from build123d import *

# Parameters (mm, degrees)
F0_R     = 1.55
F1_DEPTH = 1.5
F2_W     = 5
F2_H     = 2
F3_DEPTH = 1.5
F4_R     = 0.5
F5_DEPTH = 25
F7_DEPTH = 1.5
F8_R     = 3


with BuildPart() as f1:
    # F0 (on Right) → F1 (new body)
    with BuildSketch(Plane.YZ):
        with BuildLine():
            Line((-10, 0), (0, 0))
            Line((0, 0), (0, 30))
            Line((0, 30), (-10, 30))
            ThreePointArc((-10, 30), (-13.7334119498, 15), (-10, 0))
        make_face()
        with Locations((-10, 9.5)):
            Circle(F0_R, mode=Mode.SUBTRACT)
        with Locations((-6.5, 12.25)):
            Circle(F0_R, mode=Mode.SUBTRACT)
        with Locations((-10, 15)):
            Circle(F0_R, mode=Mode.SUBTRACT)
        with Locations((-10, 20.5)):
            Circle(F0_R, mode=Mode.SUBTRACT)
        with Locations((-6.5, 17.75)):
            Circle(F0_R, mode=Mode.SUBTRACT)
        with Locations((-3, 15)):
            Circle(F0_R, mode=Mode.SUBTRACT)
    extrude(amount=F1_DEPTH)

    # F2 (on face) → F3 (join)
    with BuildSketch(Plane.YZ.offset(1.5)):
        with Locations((-5, 31)):
            Rectangle(F2_W, F2_H)
        with Locations((-5, -1)):
            Rectangle(F2_W, F2_H)
    extrude(amount=-F3_DEPTH)

    # F4 (on face) → F5 (cut)
    with BuildSketch(Plane.YZ.offset(1.5)):
        with Locations((-8, 30)):
            Circle(F4_R)
        with Locations((-2, 30)):
            Circle(F4_R)
        with Locations((-2, 0)):
            Circle(F4_R)
        with Locations((-8, 0)):
            Circle(F4_R)
    extrude(amount=-F5_DEPTH, mode=Mode.SUBTRACT)

    # F6 (on face) → F7 (join)
    with BuildSketch(Plane.YZ.offset(1.5)):
        with BuildLine():
            Line((0, 18.0103986447), (0, 11.9896013553))
            ThreePointArc((0, 11.9896013553), (1.25, 15), (0, 18.0103986447))
        make_face()
    extrude(amount=-F7_DEPTH)

    # F8
    f8_edges = [f1.edges().sort_by_distance(p)[0] for p in [
        (0.75, 0, 11.989601),
        (0.75, 0, 18.010399),
    ]]
    fillet(f8_edges, radius=F8_R)


solid = f1.part
Build history of the part. All positions in model axes, mm. A direction names the side the tool comes from. Coordinates: 2 decimals unless noted, no trailing zeros. Order: outer loops, then holes, each group sorted by start corner. A loop starts at its lowest first (then second) coordinate and runs counter-clockwise, first axis right, second up. Notation, with made-up numbers: (75.25, -0.5) - (133.25, -0.5) arc R21 ccw to (133.25, 6.5) - close; hole circle Ø11 at (-31.75, 53.5). An arc over 180 degrees is marked (long way). Write item = value, one per line. Start each with the question number.
1) Two-plate mould, pull along Y, no slides. Class faces 1 (the face through (0.74, -3.202, 16.537)), 2 (the face through (0.74, 0.13, 11.8)), 3 (the face through (1.5, -6, 15)), 4 (the face through (0.8, -8, 0.5)): pulls with the +Y half, pulls with the -Y half, needs draft (parallel to the pull), parting line crosses it, or undercut.
2) Saw through at B-B on x = 0.25. Write the cut outline in (y, z), then the cut area to 3 significant figures.
3) Saw through at A-A on y = -6.5. Write the cut outline in (x, z).
4) Saw through at D-D on y = -3. Write the cut outline in (x, z), then the cut area to 4 significant figures.
5) Saw through at C-C on z = 15. Write the cut outline in (x, y).
6) 3-axis set-ups, long thin cutter, end or side, ignore diameter. For faces 5 (the face through (1, -1, 0)), 6 (the face through (1, -2.5, 31)), 7 (the face through (1, -9, 30)), 8 (the face through (0.74, -13.733, 15.219)): which of +Z, -Z, +X, -X, +Y, -Y reach the whole face in a straight line?
7) Wall check: line 1 along Z through (x, y) = (0.5, -6.5); line 2 along Z through (x, y) = (0.1, -10.25); line 3 along Z through (x, y) = (0.6, -8.75). Give the ranges that are in metal, low to high. Write a range as from..to.
From the geometry:
q1.face_1 = undercut
q1.face_2 = pulls with the +Y half
q1.face_3 = needs draft
q1.face_4 = undercut
q2.outline = (-10, 0) - (-8.5, 0) arc R0.5 cw to (-7.5, 0) - (-7.5, -2) - (-2.5, -2) - (-2.5, 0) arc R0.5 cw to (-1.5, 0) - (0, 0) - (0, 10.93) arc R3 cw to (0.52, 12.61) arc R4.25 ccw to (0.52, 17.39) arc R3 cw to (0, 19.07) - (0, 30) - (-1.5, 30) arc R0.5 cw to (-2.5, 30) - (-2.5, 32) - (-7.5, 32) - (-7.5, 30) arc R0.5 cw to (-8.5, 30) - (-10, 30) arc R32 ccw to start; hole circle Ø3.1 at (-10, 9.5); hole circle Ø3.1 at (-10, 15); hole circle Ø3.1 at (-10, 20.5); hole circle Ø3.1 at (-6.5, 12.25); hole circle Ø3.1 at (-6.5, 17.75); hole circle Ø3.1 at (-3, 15)
q2.area = 354 mm^2
q3.outline = (0, -2) - (1.5, -2) - (1.5, 10.7) - (0, 10.7) - close; (0, 13.8) - (1.5, 13.8) - (1.5, 16.2) - (0, 16.2) - close; (0, 19.3) - (1.5, 19.3) - (1.5, 32) - (0, 32) - close
q4.outline = (0, -2) - (1.5, -2) - (1.5, 13.45) - (0, 13.45) - close; (0, 16.55) - (1.5, 16.55) - (1.5, 32) - (0, 32) - close
q4.area = 46.35 mm^2
q5.outline = (0, -13.73) - (1.5, -13.73) - (1.5, -11.55) - (0, -11.55) - close; (0, -8.45) - (1.5, -8.45) - (1.5, -4.55) - (0, -4.55) - close; (0, -1.45) - (1.5, -1.45) - (1.5, 1.25) - (0, 1.25) - close
q6.face_5 = -Z, +X, -X, +Y
q6.face_6 = +Z, +X, -X, +Y
q6.face_7 = +Z, +X, -X, -Y
q6.face_8 = +X, -X, -Y
q7.line_1 = -2..10.7, 13.8..16.2, 19.3..32
q7.line_2 = 0.48..7.97, 11.03..13.47, 16.53..18.97, 22.03..29.52
q7.line_3 = 0..8.58, 10.42..14.08, 15.92..19.58, 21.42..30
